from build123d import *

# Parameters (mm, degrees)
SALIENTE_EXTRUIR1_DEPTH = 3
CROQUIS2_R              = 1.55
CORTAR_EXTRUIR1_DEPTH   = 3


with BuildPart() as part:
    # Model → Saliente-Extruir1 (new body)
    with BuildSketch(Plane.XY):
        Polygon((186, 103), (186, 90.195), (183, 90.195), (183, 65.805), (186, 65.805), (186, 53), (220.805, 53), (220.805, 56), (245.195, 56), (245.195, 53), (269.585, 53), (280, 53), (280, 65.805), (283, 65.805), (283, 90.195), (280, 90.195), (280, 103), align=None)
    extrude(amount=SALIENTE_EXTRUIR1_DEPTH)

    # Croquis2 → Cortar-Extruir1 (cut)
    with BuildSketch(Plane.XY.offset(3)):
        with Locations((233, 78)):
            Circle(CROQUIS2_R)
        with Locations((198, 78)):
            Circle(CROQUIS2_R)
    extrude(amount=-CORTAR_EXTRUIR1_DEPTH, mode=Mode.SUBTRACT)


solid = part.part
Could you check a few things on this model? Use its own coordinates, in mm. A direction names the side the tool comes from. Round coordinates to 2 decimals unless told otherwise and drop trailing zeros. Loops run counter-clockwise (first coordinate to the right, second up) from the corner with the lowest first, then second, coordinate; pieces in that order, holes last. Notation, with made-up numbers: (78, 14) -> (109, 14) arc R6 cw to (109, 22) -> close; hole circle Ø8 at (50.25, 62.5). An arc over 180 degrees is marked (long way). Use CSV: the item, a comma, the result in double quotes.
(1) If I drill on probe 1 along X at (y, z) = (78, 1.45); probe 2 along Y at (x, z) = (198, 1.3); probe 3 along Y at (x, z) = (233, 1.35), over which ranges is the centre line in solid material (lowest first)? Write a range as [from, to].
Return value:
probe 1,"x = [183, 196.45], [199.55, 231.45], [234.55, 283]"
probe 2,"y = [53, 76.45], [79.55, 103]"
probe 3,"y = [56, 76.45], [79.55, 103]"
(2) Suppose I cut it at D-D on x = 233. Write out the boundary of the cut face in (y, z).
Return value:
outline,"(56, 0) -> (76.45, 0) -> (76.45, 3) -> (56, 3) -> close; (79.55, 0) -> (103, 0) -> (103, 3) -> (79.55, 3) -> close"
(3) Will these pins go through, and if not, where does the flat tip stop? pin 1 Ø1.5 at (y, z) = (62, 2) entering from +X; pin 2 Ø1.5 at (x, z) = (281, 2) entering from +Y (3 decimals); pin 3 Ø5 at (x, y) = (258, 65) entering from -Z.
Return value:
pin 1,"stops at x = 280"
pin 2,"stops at y = 90.195"
pin 3,"stops at z = 0"
(4) Suppose I cut it at B-B on y = 78. Write out the boundary of the cut face in (x, z), plus the area to 3 significant figures.
Return value:
outline,"(183, 0) -> (196.45, 0) -> (196.45, 3) -> (183, 3) -> close; (199.55, 0) -> (231.45, 0) -> (231.45, 3) -> (199.55, 3) -> close; (234.55, 0) -> (283, 0) -> (283, 3) -> (234.55, 3) -> close"
area,"281 mm²"
(5) For faces 1 (the flat face through (220.805, 54, 1)), 2 (the flat face through (282, 90.195, 1)), 3 (the flat face through (281, 65.805, 1)), which set-ups out of +Z, -Z, +X, -X, +Y, -Y let a thin tool reach every point of the face, with its end or its side?
Return value:
face 1,"+Z, -Z, -Y"
face 2,"+Z, -Z, +X, +Y"
face 3,"+Z, -Z, +X, -Y"
(6) Suppose I cut it at C-C on z = 1.15. Write out the boundary of the cut face in (x, y) (3 decimals).
Return value:
outline,"(183, 65.805) -> (186, 65.805) -> (186, 53) -> (220.805, 53) -> (220.805, 56) -> (245.195, 56) -> (245.195, 53) -> (280, 53) -> (280, 65.805) -> (283, 65.805) -> (283, 90.195) -> (280, 90.195) -> (280, 103) -> (186, 103) -> (186, 90.195) -> (183, 90.195) -> close; hole circle Ø3.1 at (198, 78); hole circle Ø3.1 at (233, 78)"
(7) If we mould it in two halves opening along X, with no side actions, what happens to faces 4 (the flat face through (233, 56, 1)), 5 (the flat face through (232, 84, 0)), 6 (the flat face through (245.195, 55, 1)), 7 (the flat face through (186, 59, 1))? For each: +X half, -X half, draft (parallel to the pull), parting line (faces both ways), or undercut.
Return value:
face 4,"undercut"
face 5,"draft"
face 6,"undercut"
face 7,"-X half"
(8) Suppose I cut it at A-A on x = 198. Write out the boundary of the cut face in (y, z).
Return value:
outline,"(53, 0) -> (76.45, 0) -> (76.45, 3) -> (53, 3) -> close; (79.55, 0) -> (103, 0) -> (103, 3) -> (79.55, 3) -> close"
